Here's how the part is built. I have some questions about the finished solid (model axes, mm). Coordinates: 2 decimals unless noted, no trailing zeros. Order: outer loops, then holes, each group sorted by start corner. A loop starts at its lowest first (then second) coordinate and runs counter-clockwise, first axis right, second up. Notation, with made-up numbers: (-28.5, 61) - (22.5, 61) arc R21 ccw to (22.5, 65) - close; hole circle Ø2 at (41.5, 68.5). An arc over 180 degrees is marked (long way). Answer as CSV lines item,"result". Start each with the question number.
Item 1: I need wall thicknesses on line 1 (Z direction, x = 155.5, y = -1.9); line 2 (X direction, y = -3.4, z = -53); line 3 (Z direction, x = 223, y = -2.1). Which ranges of each line are inside material? Lowest first, please.
Item 2: Imagine slicing it at B-B on z = -50. List the corners of the cut face in (x, y) for me, and give its area (3 significant figures).
Item 3: Imagine slicing it at A-A on x = 25. List the corners of the cut face in (y, z) for me.
Item 4: Imagine slicing it at C-C on y = -3.35. List the corners of the cut face in (x, z) for me, and give its area (3 significant figures).
Item 5: I'm going to push a flat-ended pin straight in: pin 1 (12.5 mm diameter, centred on x = 25, z = -50, fed in from +Y). Where does the tip first touch, or does it pass through?
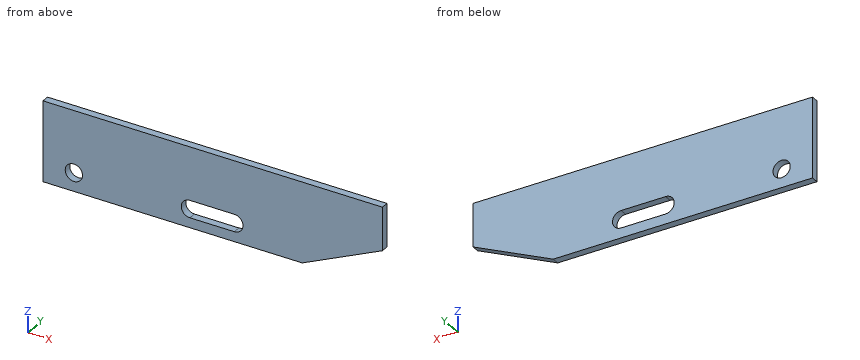
from build123d import *

# Parameters (mm, degrees)
F0_R     = 7
F1_DEPTH = 6


with BuildPart() as f1:
    # F0 (on Front) → F1 (new body)
    with BuildSketch(Plane.XZ):
        Polygon((275, 0), (0, 0), (0, -65), (210, -65), (275, -35), align=None)
        with Locations((25, -50)):
            Circle(F0_R, mode=Mode.SUBTRACT)
        with BuildLine():
            ThreePointArc((154.999536, -43), (162, -49.999783), (154.999969, -57))
            Line((154.999969, -57), (119.04693, -56.999843))
            ThreePointArc((119.04693, -56.999843), (112.000947, -50.11512), (118.816702, -43.0024))
            ThreePointArc((118.816702, -43.0024), (118.999536, -43), (119.18237, -43.002376))
            Line((119.18237, -43.002376), (154.999536, -43))
        make_face(mode=Mode.SUBTRACT)
    extrude(amount=F1_DEPTH)


solid = f1.part
Responses:
1,line 1,"z = -65 to -56.98, -43.02 to 0"
1,line 2,"x = 0 to 18.68, 31.32 to 112.68, 161.32 to 236"
1,line 3,"z = -59 to 0"
2,outline,"(0, -6) - (18, -6) - (18, 0) - (0, 0) - close; (32, -6) - (112, -6) - (112, 0) - (32, 0) - close; (162, -6) - (242.5, -6) - (242.5, 0) - (162, 0) - close"
2,area,"1,070 mm^2"
3,outline,"(-6, -65) - (0, -65) - (0, -57) - (-6, -57) - close; (-6, -43) - (0, -43) - (0, 0) - (-6, 0) - close"
4,outline,"(0, -65) - (210, -65) - (275, -35) - (275, 0) - (0, 0) - close; hole circle Ø14 at (25, -50); hole (118.82, -43) arc R7 ccw to (119.05, -57) - (155, -57) arc R7 ccw to (155, -43) - (119.18, -43) arc R7 ccw to start"
4,area,"16,100 mm^2"
5,pin 1,"passes through"
